Autodesk Fusion 360 part; units mm, degrees
sketch "Sketch1" plane through (0, 0, 0) normal (1, 0, 0) x (0, 1, 0)
  line L0 (2.8, 6) -> (2.8, 5.1079)
  arc A0 (2.8, 6) -> (-2.8, 6) centre (0, 6) ccw
  arc A1 (-2.8, 5.1079) -> (2.8, 5.1079) centre (0, 0) ccw
  line L1 (-2.8, 5.1079) -> (-2.8, 6)
  circle A2 centre (0, 0) radius 2.5
  circle A3 centre (0, 0) radius 11.25
  circle A4 centre (0, 0) radius 2.5
  line L2 (2.8, 6) -> (2.8, 5.1079)
  circle A5 centre (0, 0) radius 11.25
  line L3 (-2.8, 5.1079) -> (-2.8, 6)
  arc A6 (2.8, 6) -> (-2.8, 6) centre (0, 6) ccw
  arc A7 (-2.8, 5.1079) -> (2.8, 5.1079) centre (0, 0) ccw
  arc A8 (-2.8, 144.8079) -> (2.8, 144.8079) centre (0, 139.7) ccw
  line L4 (2.8, 145.7) -> (2.8, 144.8079)
  circle A9 centre (0, 139.7) radius 11.25
  circle A10 centre (0, 139.7) radius 11.25
  circle A11 centre (0, 139.7) radius 2.5
  line L5 (-2.8, 144.8079) -> (-2.8, 145.7)
  line L6 (2.8, 145.7) -> (2.8, 144.8079)
  circle A12 centre (0, 139.7) radius 2.5
  arc A13 (2.8, 145.7) -> (-2.8, 145.7) centre (0, 145.7) ccw
  arc A14 (2.8, 145.7) -> (-2.8, 145.7) centre (0, 145.7) ccw
  line L7 (-2.8, 144.8079) -> (-2.8, 145.7)
  arc A15 (-2.8, 144.8079) -> (2.8, 144.8079) centre (0, 139.7) ccw
  line L8 (0, 139.7) -> (0, 0) construction
  line L9 (0, 139.7) -> (-11.25, 139.7) construction
  line L10 (0, 0) -> (-11.25, 0) construction
  line L11 (0, 69.85) -> (50, 69.85) construction
  arc A16 (-7.2247, 139.7) -> (-7.2753, 140.1491) centre (-629.3846, 69.85) ccw
  arc A17 (-7.2753, -0.4491) -> (-7.2247, 0) centre (-629.3846, 69.85) ccw
  line L12 (11.25, 139.7) -> (11.25, 0)
  line L13 (-11.25, 139.7) -> (-11.25, 0)
  arc A18 (7.25, 116.7) -> (-7.25, 116.7) centre (0, 116.7) ccw
  arc A19 (-7.25, 23) -> (7.25, 23) centre (0, 23) ccw
  line L14 (-7.25, 116.7) -> (-7.25, 23)
  line L15 (7.25, 116.7) -> (7.25, 23)
  circle A20 centre (0, 128.45) radius 2.25
  circle A21 centre (0, 11.25) radius 2.25
  arc A22 (-4.25, 23) -> (4.25, 23) centre (0, 23) ccw
  line L16 (4.25, 116.7) -> (4.25, 23)
  arc A23 (4.25, 116.7) -> (-4.25, 116.7) centre (0, 116.7) ccw
  line L17 (-4.25, 116.7) -> (-4.25, 23)
  point P0 (0, 5.375)
  point P1 (0, 5.375)
  point P2 (0, 150.95)
  point P3 (0, 145.075)
  point P4 (0, 150.95)
  point P5 (0, 139.7)
  point P6 (0, 139.7)
  point P7 (0, 145.075)
  dimension "d1" = 11.65
  dimension "d3" = 5.6
  dimension "d4" = 6
  dimension "d5" = 5
  dimension "d6" = 22.5
  dimension "d8" = 11.65
  dimension "d9" = 5.6
  dimension "d10" = 6
  dimension "d11" = 5
  dimension "d12" = 22.5
  dimension "d14" = 11.65
  dimension "d15" = 5.6
  dimension "d16" = 6
  dimension "d17" = 5
  dimension "d18" = 22.5
  dimension "d19" = 11.65
  dimension "d20" = 5.6
  dimension "d21" = 6
  dimension "d22" = 5
  dimension "d23" = 22.5
  dimension "d60" = 4.5
  dimension "d63" = -3
extrude "Extrude1" add sketch "Sketch1" against normal blind 4 contours L0 A0 A1 L1 L2 L3 A6 A7 | A3 A5 A21 | A3 A5 A9 A10 L12 L13 A20 A21 | A3 A5 A21 | A3 A5 A21 | A9 A10 A20 | A9 A10 A20 | A9 A10 A20 | A8 L4 L5 L6 A13 A14 L7 A15 | A18 A19 L14 L15
ref_plane "WorkPlane1" through (25.5, 0, 69.85) normal (1, 0, 0) x (0, 1, 0)
chamfer "Chamfer1" distance 2 angle 45 8 edges at (0, 11.25, 69.85) (0, 0, -11.25) (0, -11.25, 69.85) (0, 0, 150.95) (-4, 0, 150.95) (-4, 11.25, 69.85) (-4, 0, -11.25) (-4, -11.25, 69.85)
chamfer "Chamfer3" distance 2 angle 45 8 edges at (0, 0, 120.95) (0, 4.25, 69.85) (0, 0, 18.75) (0, -4.25, 69.85) (-4, 0, 120.95) (-4, -4.25, 69.85) (-4, 0, 18.75) (-4, 4.25, 69.85)
sketch "Sketch2" plane through (25.5, 0, 0) normal (1, 0, 0) x (0, 1, 0)
  arc A0 (-2.8, 144.8079) -> (2.8, 144.8079) centre (0, 139.7) ccw
  arc A1 (2.8, 145.7) -> (-2.8, 145.7) centre (0, 145.7) ccw
  line L0 (11.25, 139.7) -> (11.25, 0)
  line L1 (0, 139.7) -> (0, 0) construction
  circle A2 centre (0, 139.7) radius 11.25
  line L2 (-2.8, 144.8079) -> (-2.8, 145.7)
  circle A3 centre (0, 139.7) radius 11.25
  line L3 (-11.25, 139.7) -> (-11.25, 0)
  circle A4 centre (0, 0) radius 11.25
  line L4 (2.8, 145.7) -> (2.8, 144.8079)
  circle A5 centre (0, 139.7) radius 2.5
  line L5 (0, 139.7) -> (-11.25, 139.7) construction
  line L6 (2.8, 145.7) -> (2.8, 144.8079)
  arc A6 (7.25, 116.7) -> (-7.25, 116.7) centre (0, 116.7) ccw
  circle A7 centre (0, 139.7) radius 2.5
  arc A8 (-7.2247, 139.7) -> (-7.2753, 140.1491) centre (-629.3846, 69.85) ccw
  arc A9 (2.8, 145.7) -> (-2.8, 145.7) centre (0, 145.7) ccw
  line L7 (-2.8, 144.8079) -> (-2.8, 145.7)
  line L8 (-7.25, 116.7) -> (-7.25, 23)
  line L9 (7.25, 116.7) -> (7.25, 23)
  arc A10 (-2.8, 144.8079) -> (2.8, 144.8079) centre (0, 139.7) ccw
  circle A11 centre (0, 0) radius 2.5
  arc A12 (2.8, 6) -> (-2.8, 6) centre (0, 6) ccw
  arc A13 (2.8, 6) -> (-2.8, 6) centre (0, 6) ccw
  line L10 (-2.8, 5.1079) -> (-2.8, 6)
  line L11 (2.8, 6) -> (2.8, 5.1079)
  circle A14 centre (0, 0) radius 2.5
  arc A15 (-2.8, 5.1079) -> (2.8, 5.1079) centre (0, 0) ccw
  arc A16 (-2.8, 5.1079) -> (2.8, 5.1079) centre (0, 0) ccw
  line L12 (2.8, 6) -> (2.8, 5.1079)
  arc A17 (-7.25, 23) -> (7.25, 23) centre (0, 23) ccw
  arc A18 (-7.2753, -0.4491) -> (-7.2247, 0) centre (-629.3846, 69.85) ccw
  circle A19 centre (0, 0) radius 11.25
  line L13 (0, 0) -> (-11.25, 0) construction
  line L14 (-2.8, 5.1079) -> (-2.8, 6)
  point P0 (0, 69.85)
  point P1 (0, 150.95)
  point P2 (0, 139.7)
  point P3 (0, 145.075)
  point P4 (0, 150.95)
  point P5 (0, 5.375)
  point P6 (0, 145.075)
  point P7 (0, 139.7)
  point P8 (0, 5.375)
  dimension "d36" = 11.65
  dimension "d37" = 5.6
  dimension "d38" = 6
  dimension "d39" = 5
  dimension "d40" = 22.5
  dimension "d41" = 11.65
  dimension "d42" = 5.6
  dimension "d43" = 6
  dimension "d44" = 5
  dimension "d45" = 22.5
  dimension "d46" = 11.65
  dimension "d47" = 5.6
  dimension "d48" = 6
  dimension "d49" = 5
  dimension "d50" = 22.5
  dimension "d51" = 11.65
  dimension "d52" = 5.6
  dimension "d53" = 6
  dimension "d54" = 5
  dimension "d55" = 22.5
  dimension "d56" = 4
  dimension "d57" = 4
extrude "Extrude2" [suppressed]
Verification items for the finished model (mm, model axes). A direction names the side the tool comes from. Coordinates: 2 decimals unless noted, no trailing zeros. Order: outer loops, then holes, each group sorted by start corner. A loop starts at its lowest first (then second) coordinate and runs counter-clockwise, first axis right, second up. Notation, with made-up numbers: M -0.5,85 L 17.5,85 A25 ccw 17.5,113 Z; hole C -12.75,67 d8. An arc over 180 degrees is marked long. Return JSON: item names as keys, results as strings.
1) Gauge pin test, flat ends, axial feed: pin 1 (1.5 mm diameter, centred on x = -2, z = 131, fed in from +Y); pin 2 (1.5 mm diameter, centred on x = -2.5, z = 38, fed in from -Y); pin 3 (2 mm diameter, centred on x = -3.5, y = 8, fed in from -Z). Record the tip position at first contact, or that the pin passes through.
Answer list:
{"pin 1": "y = 11.25", "pin 2": "y = -11.25", "pin 3": "z = -7.52"}
2) Cross-section at A-A, the plane y = 0. Count the separate pieces of the cut face and the enclosed holes in it, and give its area (3 significant figures).
Answer list:
{"separate pieces": "4", "enclosed holes": "0", "area": "184 mm2"}
3) Thickness scan on L1, parallel to Z at x = -2.3, y = 0; L2, parallel to Z at x = -2.7, y = 0; L3, parallel to Z at x = -2.35, y = -4. Record the ranges inside material, lowest first. Write a range as [from, to].
Answer list:
{"L1": "[-10.95, -2.5], [2.5, 18.45], [121.25, 137.2], [142.2, 150.65]", "L2": "[-10.55, -2.5], [2.5, 18.05], [121.65, 137.2], [142.2, 150.25]", "L3": "[-10.14, 20.73], [118.97, 149.84]"}
4) Release check for a two-part mould opening along Z. For faces 4 (the cylindrical face through (-1.97, 1.34, 141.81)), 5 (the conical face through (-3.875, 0.206, 149.073)), 6 (the flat face through (-4, -8, 71)) record: +Z half, -Z half, draft (parallel to the pull), parting line (faces both ways), or undercut.
Answer list:
{"face 4": "undercut", "face 5": "+Z half", "face 6": "draft"}
5) Cross-section at D-D, the plane x = -3.35. Record the boundary of the cut face in (y, z), and give its area (3 significant figures).
Answer list:
{"outline": "M -9.9,0 A9.9 ccw 9.9,0 L 9.9,139.7 A9.9 ccw -9.9,139.7 Z; hole M -5.6,23 A5.6 ccw 5.6,23 L 5.6,116.7 A5.6 ccw -5.6,116.7 Z; hole C 0,0 d5; hole C 0,139.7 d5", "area": "1,890 mm2"}
6) Access from +Z, -Z, +X, -X, +Y, -Y to the whole of each face (thin tool, end or side, straight path). Record for faces 1 (the conical face through (-2.125, 0.096, 18.626)), 2 (the conical face through (-0.125, -0.206, 149.073)), 3 (the conical face through (-1.875, 0.096, 121.074)).
Answer list:
{"face 1": "-X", "face 2": "+Z, +X", "face 3": "+X"}
